Could you check a few things on this model? Use its own coordinates, in mm. A direction names the side the tool comes from. Give positions to 0.01 mm unless a question says otherwise; leave off trailing zeros. Order: outer loops, then holes, each group sorted by start corner. A loop starts at its lowest first (then second) coordinate and runs counter-clockwise, first axis right, second up. Notation, with made-up numbers: (41, 75) -> (64, 75) arc R26 cw to (64, 101) -> close; hole circle Ø2 at (73.25, 88). An arc over 180 degrees is marked (long way). Use one line per item in the form item = value. Start each with the question number.
from build123d import *

# Parameters (mm, degrees)
F0_W           = 65.687917
F0_H           = 65.738029
F1_DEPTH       = 76.2
F3_D           = 6.35
F3_CSINK_D     = 12.7
F3_CSINK_ANGLE = 90
F5_D           = 12.7
F5_CBORE_D     = 25.4
F5_CBORE_DEPTH = 12.7


with BuildPart() as f1:
    # F0 (on Right) → F1 (new body)
    with BuildSketch(Plane.YZ):
        with Locations((6.479423, -2.465733)):
            Rectangle(F0_W, F0_H)
    extrude(amount=F1_DEPTH)

    # F3 (through all)
    with Locations(Plane.YZ.offset(76.2)):
        with Locations((-6.490372, 9.031592), (18.086735, 7.191747)):
            CounterSinkHole(F3_D / 2, F3_CSINK_D / 2, counter_sink_angle=F3_CSINK_ANGLE)

    # F5 (through all)
    with Locations(Plane.XZ.offset(26.364535)):
        with Locations((54.363161, 15.718481), (54.363161, -22.743117)):
            CounterBoreHole(F5_D / 2, F5_CBORE_D / 2, F5_CBORE_DEPTH)


solid = f1.part
(1) Imagine slicing it at C-C (z = 20.5). Write out the boundary of the cut face in (x, y).
(2) Which directions (+Z, -Z, +X, -X, +Y, -Y) give clear straight access to the entire face, cutting with the end or side of a thin tool? Please do faces 1 (the cylindrical face through (66.477, -20.103, 19.533)), 2 (the cylindrical face through (51.433, 13.2, -28.377)).
(3) We'd pull the mould along Y, two halves only. Please class faces 3 (the conical face through (73.2, -9.7, 10)), 4 (the cylindrical face through (54.898, -20.103, -10.054)), 5 (the flat face through (48.5, -13.665, -19.7)): pulls with the +Y half, pulls with the -Y half, needs draft (parallel to the pull), parting line crosses it, or undercut.
(4) Imagine slicing it at B-B (y = 28). Write out the boundary of the cut face in (x, z).
(5) I'm going to push a flat-ended pin straight in: pin 1 Ø20.5 at (x, z) = (54.36, 15.72) entering from -Y. Where does the tip first touch, or does it pass through?
(6) Imagine slicing it at A-A (z = -24.5). Write out the boundary of the cut face in (x, y).
(7) Please list where these lines run through material, in increasing order: probe 1 along Z at (x, y) = (60, -18); probe 2 along Z at (x, y) = (43.5, -22); probe 3 along X at (y, z) = (-15, -12).
Calculated:
q1.outline = (0, -26.36) -> (42.6, -26.36) -> (42.6, -13.66) -> (50.18, -13.66) -> (50.18, 39.32) -> (0, 39.32) -> close; (58.54, -13.66) -> (66.13, -13.66) -> (66.13, -26.36) -> (76.2, -26.36) -> (76.2, 39.32) -> (58.54, 39.32) -> close
q2.face_1 = -Y
q2.face_2 = +Y, -Y
q3.face_3 = undercut
q3.face_4 = needs draft
q3.face_5 = pulls with the -Y half
q4.outline = (0, -35.33) -> (76.2, -35.33) -> (76.2, 30.4) -> (0, 30.4) -> close; hole circle Ø12.7 at (54.36, -22.74); hole circle Ø12.7 at (54.36, 15.72)
q5.pin_1 = -13.66
q6.outline = (0, -26.36) -> (41.79, -26.36) -> (41.79, -13.66) -> (48.26, -13.66) -> (48.26, 39.32) -> (0, 39.32) -> close; (60.47, -13.66) -> (66.94, -13.66) -> (66.94, -26.36) -> (76.2, -26.36) -> (76.2, 39.32) -> (60.47, 39.32) -> close
q7.probe_1 = -35.33 to -34.12, -11.36 to 4.34, 27.1 to 30.4
q7.probe_2 = -35.33 to -29.32, -16.16 to 9.14, 22.3 to 30.4
q7.probe_3 = 0 to 47.59, 61.14 to 76.2
